```python
from build123d import *

# Parameters (mm, degrees)
F0_R     = 60
F0_R_2   = 80
F1_DEPTH = 15


with BuildPart() as f1:
    # F0 (on Front) → F1 (new body, symmetric)
    with BuildSketch(Plane.XZ):
        with BuildLine():
            Line((360, 449), (-360, 449))
            Line((-360, 449), (-360, 219))
            Line((-360, 219), (-79.719446, -75.794524))
            ThreePointArc((-79.719446, -75.794524), (0, -110), (79.719446, -75.794524))
            Line((79.719446, -75.794524), (360, 219))
            Line((360, 219), (360, 449))
        make_face()
        Circle(F0_R, mode=Mode.SUBTRACT)
        with Locations((-225, 349)):
            Circle(F0_R_2, mode=Mode.SUBTRACT)
        with Locations((225, 349)):
            Circle(F0_R_2, mode=Mode.SUBTRACT)
    extrude(amount=F1_DEPTH, both=True)


solid = f1.part
```
Input: part model. Units: mm. Frame: model coordinates. Round coordinates to 2 decimals unless told otherwise and drop trailing zeros. Loops run counter-clockwise (first coordinate to the right, second up) from the corner with the lowest first, then second, coordinate; pieces in that order, holes last. Notation, with made-up numbers: (44.25, -37.5) -> (55.25, -37.5) arc R20 ccw to (55.25, 0.5) -> close; hole circle Ø4 at (-25.75, 32). An arc over 180 degrees is marked (long way). One line per item, written item: value.
(1) Section B-B (y = -6.25). Return the cut outline in (x, z).
Geometry check:
outline: (-360, 219) -> (-79.72, -75.79) arc R110 ccw to (79.72, -75.79) -> (360, 219) -> (360, 449) -> (-360, 449) -> close; hole circle Ø160 at (-225, 349); hole circle Ø120 at (0, 0); hole circle Ø160 at (225, 349)
(2) Section D-D (z = 0). Return the cut outline in (x, y), plus the area to 3 significant figures.
Geometry check:
outline: (-151.78, -15) -> (-60, -15) -> (-60, 15) -> (-151.78, 15) -> close; (60, -15) -> (151.78, -15) -> (151.78, 15) -> (60, 15) -> close
area: 5,510 mm2
(3) Pin query (flat end, axial travel): pin 1 (8 mm diameter, centred on y = 7.5, z = -42.5, fed in from +X); pin 2 (1 mm diameter, centred on y = -4.5, z = 141.5, fed in from +X); pin 3 (1 mm diameter, centred on y = 10, z = 166.5, fed in from -X). Return the tip coordinate at first contact, or that it passes through.
Geometry check:
pin 1: x = 115.18
pin 2: x = 286.79
pin 3: x = -310.56
(4) Section C-C (x = 0). Return the cut outline in (y, z), plus the area to 3 significant figures.
Geometry check:
outline: (-15, -110) -> (15, -110) -> (15, -60) -> (-15, -60) -> close; (-15, 60) -> (15, 60) -> (15, 449) -> (-15, 449) -> close
area: 13,200 mm2
(5) Mould query, pull axis X, two halves, no side actions, for faces 1 (the face through (-221.822, -0.21, 73.666)), 2 (the face through (261.92, 0.21, 278.03)), 3 (the face through (-1.248, -0.21, -109.993)), 4 (the face through (-5, -15, 236)). Classes: pulls with the +X half, pulls with the -X half, needs draft (parallel to the pull), parting line crosses it, or undercut.
Geometry check:
face 1: pulls with the -X half
face 2: undercut
face 3: parting line crosses it
face 4: needs draft
(6) Material intervals for line 1 (Z direction, x = 0, y = 5.25); line 2 (X direction, y = 6.25, z = 361); line 3 (Z direction, x = 234.5, y = 6.25), sorted ascending. Write a range as [from, to].
Geometry check:
line 1: [-110, -60], [60, 449]
line 2: [-360, -304.09], [-145.91, 145.91], [304.09, 360]
line 3: [87, 269.57], [428.43, 449]
(7) Section A-A (z = 349). Return the cut outline in (x, y), plus the area to 3 significant figures.
Geometry check:
outline: (-360, -15) -> (-305, -15) -> (-305, 15) -> (-360, 15) -> close; (-145, -15) -> (145, -15) -> (145, 15) -> (-145, 15) -> close; (305, -15) -> (360, -15) -> (360, 15) -> (305, 15) -> close
area: 12,000 mm2
